Answer from the drawing. Dimensions are ordinates in mm from the lowest x, y and z of the part. A direction names the side the tool comes from. Round coordinates to 2 decimals unless told otherwise and drop trailing zeros. Write each loop counter-clockwise with the first axis right and the second up, starting at its lowest first coordinate (ties: lowest second). Pieces come first, ordered by that corner, then holes.
1. Find section A-A (z = 6). Write down the section's boundary in (x, y).
2. A tool of negligible diameter and unlimited length cuts with its end or side. For the marked faces 1, 2 and 3, from which of +Z, -Z, +X, -X, +Y, -Y can it reach the whole face along a straight path? Write none if from no direction.
3. Flat-ended cylindrical pins translate along their axes: pin 1 Ø1.5 at (x, z) = (10, 1) entering from -Y; pin 2 Ø1 at (x, z) = (10, 7) entering from +Y (1 decimal). Find the tip coordinate at first contact, or state that the pin passes through.
4. Determine the mould class of the marked faces 4, 5 and 6 for opening direction X: pulls with the +X half, pulls with the -X half, needs draft (parallel to the pull), parting line crosses it, or undercut.
5. Straight lines are drawn through the part: probe 1 along Z at (x, y) = (4, 7.5); probe 2 along Z at (x, y) = (2.5, 1.5) (1 decimal); probe 3 along X at (y, z) = (6.75, 3.5) (1 decimal). For each, find the intervals that lie inside material, in ascending order.
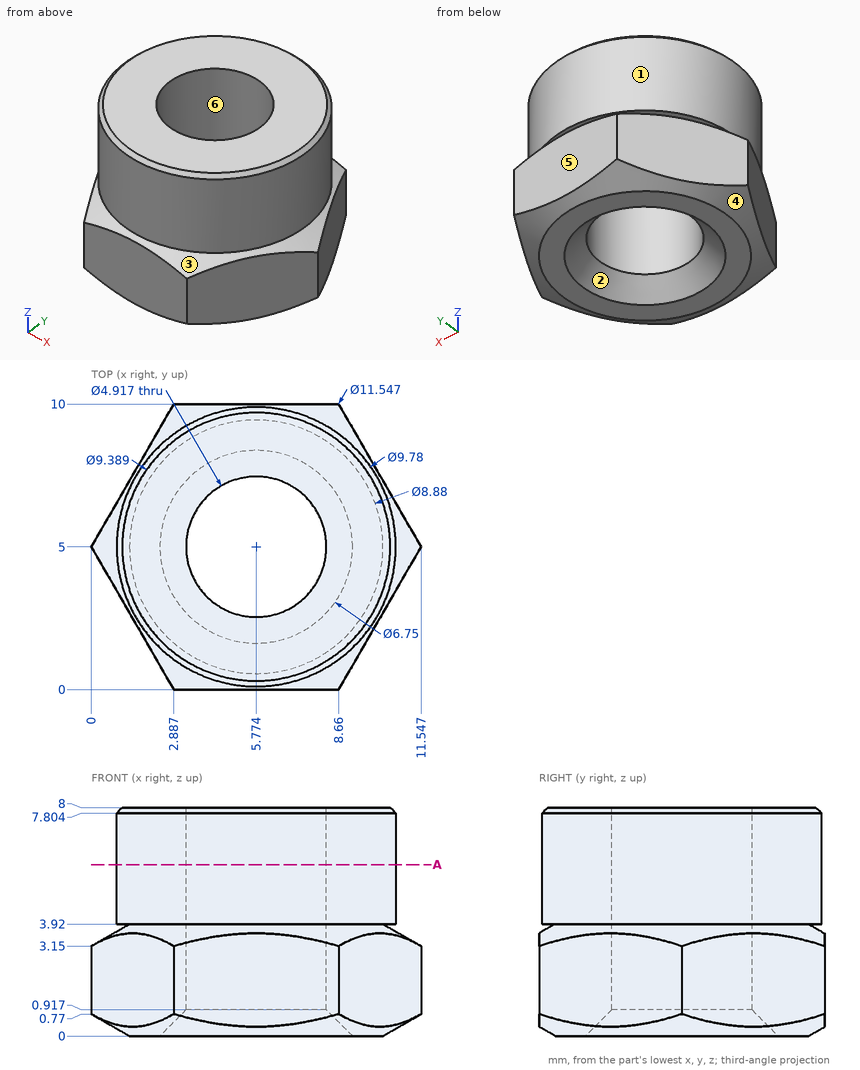
Worked answers:
1. outline: circle Ø9.78 at (5.77, 5); hole circle Ø4.92 at (5.77, 5)
2. face 1: +Z
2. face 2: -Z
2. face 3: none
3. pin 1: stops at y = 1.02
3. pin 2: stops at y = 8.2
4. face 4: parting line crosses it
4. face 5: needs draft
4. face 6: undercut
5. probe 1: z = 0.31 to 8
5. probe 2: z = 0.2 to 3.7, 3.9 to 7.9
5. probe 3: x = 1 to 4, 7.5 to 10.5
